Build history of the part. All positions in model axes, mm. A direction names the side the tool comes from. Coordinates: 2 decimals unless noted, no trailing zeros. Loops run counter-clockwise (first coordinate to the right, second up) from the corner with the lowest first, then second, coordinate; pieces in that order, holes last.
(1) Two-plate mould, pull along Z, no slides. Class faces 4 (the face through (-53.574, -41.421, 36.975)), 5 (the face through (-25, 29, 0)), 6 (the face through (39.8, -26.21, 63.2)): pulls with the +Z half, pulls with the -Z half, needs draft (parallel to the pull), parting line crosses it, or undercut.
(2) Slice it at D-D (y = -33). Give the cut face in (x, z).
(3) Wall check: L1, parallel to Y at x = -34.75, z = 55.5 (3 decimals); L2, parallel to Y at x = 0, z = 38 (3 decimals); L3, parallel to Y at x = -25.5, z = 50.5 (3 decimals). Give the ranges that are in metal, low to high.
(4) Slice it at C-C (z = 18). Give the cut face in (x, y) (3 decimals), and give its area (3 significant figures).
(5) Flat gauge pin, fed straight in: P1, Ø4, axis at x = -34.75, y = 34.745, coming from the +Z side. Where does the tip first touch, or does it go through?
(6) Slice it at A-A (y = 0). Give the number of separate pieces and of enclosed holes in the cut face, and give its area (3 significant figures).
(7) Slice it at B-B (x = 0). Give the cut face in (y, z) (3 decimals), and give its area (3 significant figures).
(8) Tool access for faces 1 (the face through (43.875, 0.22, 4.93)), 2 (the face through (53.574, 41.421, 36.975)), 3 (the face through (-43, 0, 10)): list every direction of +Z, -Z, +X, -X, +Y, -Y with a clear straight run to the whole face (end or side of a thin tool).
from build123d import *

# Parameters (mm, degrees)
F0_R          = 3.25
F0_R_2        = 5
F0_R_3        = 37.5
F0_R_4        = 3
F1_DEPTH      = 75
F3_DEPTH      = 129.5235
F3_DEPTH_BACK = 58.3597
F4_DEPTH      = 40.69625


with BuildPart() as f1:
    # F0 (on Top) → F1 (new body)
    with BuildSketch(Plane.XY):
        with BuildLine():
            Line((50, 42.925), (-50, 42.925))
            ThreePointArc((-50, 42.925), (-53.535534, 41.460534), (-55, 37.925))
            Line((-55, 37.925), (-55, -37.925))
            ThreePointArc((-55, -37.925), (-53.535534, -41.460534), (-50, -42.925))
            Line((-50, -42.925), (50, -42.925))
            ThreePointArc((50, -42.925), (53.535534, -41.460534), (55, -37.925))
            Line((55, -37.925), (55, 37.925))
            ThreePointArc((55, 37.925), (53.535534, 41.460534), (50, 42.925))
        make_face()
        with Locations((-34.75, -34.745)):
            Circle(F0_R, mode=Mode.SUBTRACT)
        with Locations((34.75, -34.745)):
            Circle(F0_R, mode=Mode.SUBTRACT)
        with Locations((-48.88, 0)):
            Circle(F0_R_2, mode=Mode.SUBTRACT)
        with Locations((-34.75, 34.745)):
            Circle(F0_R, mode=Mode.SUBTRACT)
        Circle(F0_R_3, mode=Mode.SUBTRACT)
        with Locations((48.87, 0)):
            Circle(F0_R_2, mode=Mode.SUBTRACT)
        with Locations((34.75, 34.745)):
            Circle(F0_R, mode=Mode.SUBTRACT)
        with Locations((48.87, 0)):
            Circle(F0_R_2)
        with Locations((48.87, 0)):
            Circle(F0_R_4, mode=Mode.SUBTRACT)
        with Locations((-48.88, 0)):
            Circle(F0_R_2)
        with Locations((-48.88, 0)):
            Circle(F0_R_4, mode=Mode.SUBTRACT)
    extrude(amount=F1_DEPTH)

    # F2 (on face) → F3 (cut, two sides)
    with BuildSketch(Plane(origin=(-55, 0, 0), x_dir=(0, -1, 0), z_dir=(-1, 0, 0))) as f3_sk:
        with BuildLine():
            Line((21.925, 65), (-21.925, 65))
            ThreePointArc((-21.925, 65), (-26.167641, 63.242641), (-27.925, 59))
            Line((-27.925, 59), (-27.925, 16))
            ThreePointArc((-27.925, 16), (-26.167641, 11.757359), (-21.925, 10))
            Line((-21.925, 10), (21.925, 10))
            ThreePointArc((21.925, 10), (26.167641, 11.757359), (27.925, 16))
            Line((27.925, 16), (27.925, 59))
            ThreePointArc((27.925, 59), (26.167641, 63.242641), (21.925, 65))
        make_face()
    extrude(amount=-F3_DEPTH, mode=Mode.SUBTRACT)
    extrude(f3_sk.sketch, amount=-F3_DEPTH_BACK, mode=Mode.SUBTRACT)

    # F0 (on Top) → F4 (cut)
    with BuildSketch(Plane.XY):
        with Locations((-48.88, 0)):
            Circle(F0_R_2)
        with Locations((-48.88, 0)):
            Circle(F0_R_4, mode=Mode.SUBTRACT)
        with Locations((48.87, 0)):
            Circle(F0_R_2)
        with Locations((48.87, 0)):
            Circle(F0_R_4, mode=Mode.SUBTRACT)
    extrude(amount=F4_DEPTH, mode=Mode.SUBTRACT)


solid = f1.part
Response values:
1. face 4: needs draft
1. face 5: pulls with the -Z half
1. face 6: undercut
2. outline: (-55, 0) - (-37.49, 0) - (-37.49, 75) - (-55, 75) - close; (-32.01, 0) - (-17.81, 0) - (-17.81, 75) - (-32.01, 75) - close; (17.81, 0) - (32.01, 0) - (32.01, 75) - (17.81, 75) - close; (37.49, 0) - (55, 0) - (55, 75) - (37.49, 75) - close
3. L1: y = -42.925 to -37.995, -31.495 to -27.925, 27.925 to 31.495, 37.995 to 42.925
3. L2: y = -42.925 to -37.5, 37.5 to 42.925
3. L3: y = -42.925 to -27.925, 27.925 to 42.925
4. outline: (-55, -37.925) arc R5 ccw to (-50, -42.925) - (50, -42.925) arc R5 ccw to (55, -37.925) - (55, -27.925) - (25.029, -27.925) arc R37.5 cw to (-25.029, -27.925) - (-55, -27.925) - close; (-55, 27.925) - (-25.029, 27.925) arc R37.5 cw to (25.029, 27.925) - (55, 27.925) - (55, 37.925) arc R5 ccw to (50, 42.925) - (-50, 42.925) arc R5 ccw to (-55, 37.925) - close; hole circle Ø6.5 at (-34.75, -34.745); hole circle Ø6.5 at (-34.75, 34.745); hole circle Ø6.5 at (34.75, -34.745); hole circle Ø6.5 at (34.75, 34.745)
4. area: 2,490 mm2
5. P1: passes through
6. separate pieces: 8
6. enclosed holes: 0
6. area: 380 mm2
7. outline: (-42.925, 0) - (-37.5, 0) - (-37.5, 75) - (-42.925, 75) - close; (37.5, 0) - (42.925, 0) - (42.925, 75) - (37.5, 75) - close
7. area: 814 mm2
8. face 1: -Z
8. face 2: +Z, -Z, +X, +Y
8. face 3: +X, -X
